The listing builds one solid part. Answer for the finished solid, in the listing's coordinates (mm). A direction names the side the tool comes from. Coordinates: 2 decimals unless noted, no trailing zeros. Order: outer loops, then holes, each group sorted by start corner. A loop starts at its lowest first (then second) coordinate and runs counter-clockwise, first axis right, second up.
```python
from build123d import *

# Parameters (mm, degrees)
F0_W     = 406.4
F0_H     = 647.7
F1_DEPTH = 152.4
F2_W     = 416.56
F2_H     = 289.56
F2_W_2   = 406.4
F2_H_2   = 152.4
F3_DEPTH = 12.7
F4_W     = 381
F4_H     = 635
F5_DEPTH = 146.05


with BuildPart() as f1:
    # F0 (on Top) → F1 (new body)
    with BuildSketch(Plane.XY):
        with Locations((203.2, -323.85)):
            Rectangle(F0_W, F0_H)
    extrude(amount=F1_DEPTH)

    # F2 (on face) → F3 (join)
    with BuildSketch(Plane.XZ.offset(647.7)):
        with Locations((203.2, 132.08)):
            Rectangle(F2_W, F2_H)
        with Locations((203.2, 76.2)):
            Rectangle(F2_W_2, F2_H_2, mode=Mode.SUBTRACT)
        with Locations((203.2, 76.2)):
            Rectangle(F2_W_2, F2_H_2)
    extrude(amount=F3_DEPTH)

    # F4 (on face) → F5 (cut)
    with BuildSketch(Plane.XY.offset(152.4)):
        with Locations((203.2, -330.2)):
            Rectangle(F4_W, F4_H)
    extrude(amount=-F5_DEPTH, mode=Mode.SUBTRACT)


solid = f1.part
```
1) A cutting plane is placed at D-D, the plane z = 184. Write down the section's boundary in (x, y).
2) Straight lines are drawn through the part: probe 1 along Y at (x, z) = (189.5, 109); probe 2 along X at (y, z) = (-179, 59); probe 3 along Z at (x, y) = (36, -589). For each, find the intervals that lie inside material, in ascending order.
3) Each of these flat-tipped pins is pushed along its axis until it touches: P1, Ø5, axis at y = -227, z = 22, coming from the +X side; P2, Ø12, axis at x = 139.5, y = -557.5, coming from the +Z side; P3, Ø4, axis at x = 203.5, z = 234, coming from the +Y side. Where does it stop, or does it pass through?
4) A cutting plane is placed at A-A, the plane z = 93. Write down the section's boundary in (x, y), plus the area to 3 significant figures.
5) A cutting plane is placed at C-C, the plane y = -548. Write down the section's boundary in (x, z).
6) The mould has two halves that part along X. Classify faces 1 (the flat face through (201, -326, 6.35)), 2 (the flat face through (0, -328, 75)), 3 (the flat face through (200, -660.4, 134)): released by +X, released by -X, zero draft, split by the parting line, or undercut.
7) For faces 4 (the flat face through (398, -226, 152.4)), 5 (the flat face through (393.7, -335, 80)), 6 (the flat face through (406.4, -328, 75)), determine the directions among +Z, -Z, +X, -X, +Y, -Y from which every point of the face is accessible in a straight line to the end or side of a thin tool.
8) A cutting plane is placed at B-B, the plane x = 34. Write down the section's boundary in (y, z).
Working result:
1. outline: (-5.08, -660.4) - (411.48, -660.4) - (411.48, -647.7) - (-5.08, -647.7) - close
2. probe 1: y = -660.4 to -647.7, -12.7 to 0
2. probe 2: x = 0 to 12.7, 393.7 to 406.4
2. probe 3: z = 0 to 6.35
3. P1: stops at x = 406.4
3. P2: stops at z = 6.35
3. P3: stops at y = -647.7
4. outline: (-5.08, -660.4) - (411.48, -660.4) - (411.48, -647.7) - (406.4, -647.7) - (406.4, 0) - (0, 0) - (0, -647.7) - (-5.08, -647.7) - close; hole (12.7, -647.7) - (393.7, -647.7) - (393.7, -12.7) - (12.7, -12.7) - close
4. area: 26,600 mm2
5. outline: (0, 0) - (406.4, 0) - (406.4, 152.4) - (393.7, 152.4) - (393.7, 6.35) - (12.7, 6.35) - (12.7, 152.4) - (0, 152.4) - close
6. face 1: undercut
6. face 2: released by -X
6. face 3: zero draft
7. face 4: +Z, +X, -X, +Y
7. face 5: +Z
7. face 6: +Z, -Z, +X, +Y
8. outline: (-660.4, -12.7) - (-647.7, -12.7) - (-647.7, 0) - (0, 0) - (0, 152.4) - (-12.7, 152.4) - (-12.7, 6.35) - (-647.7, 6.35) - (-647.7, 276.86) - (-660.4, 276.86) - close
